Source: CAD feature listing. Evaluate the final solid. Frame: model axes, mm. A direction names the side the tool comes from. Give positions to 0.01 mm unless a question says otherwise; leave off trailing zeros. Write each loop counter-clockwise with the first axis right and the second up, starting at its lowest first coordinate (ties: lowest second). Pieces come first, ordered by that corner, then holes. Notation, with made-up numbers: (21, 24.25) -> (29, 24.25) arc R17 ccw to (29, 31.25) -> close; hole circle Ø5 at (44.25, 74). An arc over 180 degrees is marked (long way). Use one line per item in the form item = value. Start each with the question number.
(1) Cut plane C-C, the plane x = -8. Output: boundary loops of the cut face in (y, z).
(2) First-contact query: P1, Ø3, axis at x = -3, y = 8.5, coming from the +Z side; P2, Ø2, axis at x = -8, z = 0, coming from the -Y side; P3, Ø3.5, axis at x = 1, z = -0.5, coming from the +Y side. Flat tips, straight axial feed; report the tip coordinate or a pass-through.
(3) Draft query along Z for faces 6 (the face through (9.25, 2.46, 0.05)), 7 (the face through (-8, 5, 0)), 8 (the face through (0, 3, 10.75)), 9 (the face through (-12.5, 2.5, -0.2)). Return one class per face: pulls with the +Z half, pulls with the -Z half, needs draft (parallel to the pull), parting line crosses it, or undercut.
(4) Cut plane A-A, the plane z = 0. Output: boundary loops of the cut face in (x, y).
(5) Cut plane B-B, the plane y = 7.5. Output: boundary loops of the cut face in (x, z).
(6) Material intervals for line 1 along Z through (x, y) = (0, 11.5); line 2 along Y through (x, z) = (2, 2); line 3 along Y through (x, z) = (8.5, 7.25), sorted ascending. Write a range as from..to.
(7) Cut plane D-D, the plane z = -6. Output: boundary loops of the cut face in (x, y).
(8) Set-up query: faces 1 (the face through (8, 5, 0)), 2 (the face through (12.5, 2.5, 0.2)), 3 (the face through (-11, 5, 0)), 4 (the face through (11, 5, 0)), 5 (the face through (0, 2, 0)). Return all of +Z, -Z, +X, -X, +Y, -Y with unobstructed straight access to the full face (end or side cutting, diameter ignored); none if empty.
from build123d import *

# Parameters (mm, degrees)
SKETCH1_R           = 12.5
BOSS_EXTRUDE1_DEPTH = 17
SKETCH2_R           = 3.5
CUT_EXTRUDE1_DEPTH  = 15
SKETCH4_OUTSIDE_W   = 34.846
SKETCH4_OUTSIDE_H   = 34.846
SKETCH4_OUTSIDE_R   = 10
CUT_EXTRUDE3_DEPTH  = 12
SKETCH5_R           = 1.25
CUT_EXTRUDE4_DEPTH  = 10
SKETCH8_R           = 10.75
SKETCH8_R_2         = 4
BOSS_EXTRUDE3_DEPTH = 9
SKETCH7_W           = 22.925756412
SKETCH7_H           = 4.884412095
CUT_EXTRUDE6_DEPTH  = 6


with BuildPart() as part:
    # Sketch1 → Boss-Extrude1 (new body)
    with BuildSketch(Plane(origin=(0, 0, 0), x_dir=(1, 0, 0), z_dir=(0, 1, 0))):
        Circle(SKETCH1_R)
    extrude(amount=BOSS_EXTRUDE1_DEPTH)

    # Sketch2 → Cut-Extrude1 (cut)
    with BuildSketch(Plane(origin=(0, 17, 0), x_dir=(1, 0, 0), z_dir=(0, 1, 0))):
        Circle(SKETCH2_R)
    extrude(amount=-CUT_EXTRUDE1_DEPTH, mode=Mode.SUBTRACT)

    # Sketch4 outside → Cut-Extrude3 (cut)
    with BuildSketch(Plane(origin=(0, 17, 0), x_dir=(1, 0, 0), z_dir=(0, 1, 0))):
        Rectangle(SKETCH4_OUTSIDE_W, SKETCH4_OUTSIDE_H)
        Circle(SKETCH4_OUTSIDE_R, mode=Mode.SUBTRACT)
    extrude(amount=-CUT_EXTRUDE3_DEPTH, mode=Mode.SUBTRACT)

    # Sketch5 → Cut-Extrude4 (cut)
    with BuildSketch(Plane.XZ):
        with Locations((-8, 0)):
            Circle(SKETCH5_R)
    cut_extrude4 = extrude(amount=-CUT_EXTRUDE4_DEPTH, mode=Mode.SUBTRACT)

    # Mirror2: Cut-Extrude4 across plane
    add(cut_extrude4.mirror(Plane(origin=(0, 0, 0), x_dir=(0, 0, 1), z_dir=(1, 0, 0))), mode=Mode.SUBTRACT)

    # Sketch8 → Boss-Extrude3 (add)
    with BuildSketch(Plane(origin=(0, 5, 0), x_dir=(1, 0, 0), z_dir=(0, 1, 0))):
        Circle(SKETCH8_R)
        Circle(SKETCH8_R_2, mode=Mode.SUBTRACT)
    extrude(amount=BOSS_EXTRUDE3_DEPTH)

    # Sketch7 → Cut-Extrude6 (cut, through all)
    with BuildSketch(Plane(origin=(0, 5, 0), x_dir=(1, 0, 0), z_dir=(0, 1, 0))):
        with Locations((0.376120232, 13.192206048)):
            Rectangle(SKETCH7_W, SKETCH7_H)
    cut_extrude6 = extrude(amount=-CUT_EXTRUDE6_DEPTH, mode=Mode.SUBTRACT)

    # Mirror3: Cut-Extrude6 across plane
    add(cut_extrude6.mirror(Plane.XY), mode=Mode.SUBTRACT)


solid = part.part
Geometry says:
q1.outline = (0, -9.6) -> (5, -9.6) -> (5, -7.18) -> (14, -7.18) -> (14, -6) -> (17, -6) -> (17, 6) -> (14, 6) -> (14, 7.18) -> (5, 7.18) -> (5, 9.6) -> (0, 9.6) -> (0, 1.25) -> (5, 1.25) -> (5, -1.25) -> (0, -1.25) -> close
q2.P1 = 10.64
q2.P2 = 5
q2.P3 = 2
q3.face_6 = undercut
q3.face_7 = undercut
q3.face_8 = pulls with the +Z half
q3.face_9 = parting line crosses it
q4.outline = (-12.5, 0) -> (-9.25, 0) -> (-9.25, 5) -> (-6.75, 5) -> (-6.75, 0) -> (6.75, 0) -> (6.75, 5) -> (9.25, 5) -> (9.25, 0) -> (12.5, 0) -> (12.5, 5) -> (10.75, 5) -> (10.75, 14) -> (10, 14) -> (10, 17) -> (3.5, 17) -> (3.5, 2) -> (-3.5, 2) -> (-3.5, 17) -> (-10, 17) -> (-10, 14) -> (-10.75, 14) -> (-10.75, 5) -> (-12.5, 5) -> close
q5.outline = circle Ø21.5 at (0, 0); hole circle Ø7 at (0, 0)
q6.line_1 = -10.75..-3.5, 3.5..10.75
q6.line_2 = 0..2
q6.line_3 = 0..5
q7.outline = (-10.97, 0) -> (10.97, 0) -> (10.97, 5) -> (8.92, 5) -> (8.92, 14) -> (8, 14) -> (8, 17) -> (-8, 17) -> (-8, 14) -> (-8.92, 14) -> (-8.92, 5) -> (-10.97, 5) -> close
q8.face_1 = -Y
q8.face_2 = +X, +Y, -Y
q8.face_3 = -X, +Y
q8.face_4 = +X, +Y
q8.face_5 = +Y
